from build123d import *

# Parameters (mm, degrees)
BOSS_EXTRUDE1_DEPTH            = 5
SKETCH3_W                      = 21
SKETCH3_H                      = 20
BOSS_EXTRUDE2_DEPTH            = 5
F_4_0MM_DOWEL_HOLE1_AT_2_COUNT = 2
F_4_0MM_DOWEL_HOLE1_AT_2_PITCH = 10
SKETCH15_W                     = 20
SKETCH15_H                     = 15
BOSS_EXTRUDE6_DEPTH            = 60
SKETCH16_W                     = 20
SKETCH16_H                     = 10
BOSS_EXTRUDE7_DEPTH            = 10


with BuildPart() as part:
    # Sketch2 → Boss-Extrude1 (new body)
    with BuildSketch(Plane(origin=(0, 0, 0), x_dir=(1, 0, 0), z_dir=(0, 1, 0))):
        Polygon((-80, -10), (-10, -10), (-10, -80), (10, -80), (10, -10), (80, -10), (80, 10), (10, 10), (10, 80), (-10, 80), (-10, 10), (-80, 10), align=None)
    extrude(amount=BOSS_EXTRUDE1_DEPTH)

    # Sketch3 → Boss-Extrude2 (add)
    with BuildSketch(Plane(origin=(0, 5, 0), x_dir=(1, 0, 0), z_dir=(0, 1, 0))):
        with Locations((-69.5, 0)):
            Rectangle(SKETCH3_W, SKETCH3_H)
    boss_extrude2 = extrude(amount=BOSS_EXTRUDE2_DEPTH)

    # Sketch5 → Ø4.0mm Dowel Hole1 (revolve, cut)
    with BuildSketch(Plane(origin=(-64.5, 10, 0), x_dir=(0, 0, 1), z_dir=(1, 0, 0))):
        Polygon((0, 0), (0, 118.830821238), (2, 117.6291), (2, 0), align=None)
    f_4_0mm_dowel_hole1 = revolve(axis=Axis((-64.5, 16.35, 0), (0, -1, 0)), mode=Mode.SUBTRACT)

    # Ø4.0mm Dowel Hole1 at 2: Ø4.0mm Dowel Hole1 ×2
    with Locations(*[(-i * F_4_0MM_DOWEL_HOLE1_AT_2_PITCH, 0, 0) for i in range(1, F_4_0MM_DOWEL_HOLE1_AT_2_COUNT)]):
        add(f_4_0mm_dowel_hole1, mode=Mode.SUBTRACT)

    # Mirror1: Boss-Extrude2, Ø4.0mm Dowel Hole1 across plane
    add(boss_extrude2.mirror(Plane(origin=(0, 0, 0), x_dir=(0, 0, 1), z_dir=(1, 0, 0))))
    add(f_4_0mm_dowel_hole1.mirror(Plane(origin=(0, 0, 0), x_dir=(0, 0, 1), z_dir=(1, 0, 0))), mode=Mode.SUBTRACT)

    # Mirror1 copy 1 sketch → Mirror1 copy 1 (revolve, cut)
    with BuildSketch(Plane(origin=(74.5, 10, 0), x_dir=(0, 0, 1), z_dir=(-1, 0, 0))):
        Polygon((0, 0), (0, -118.830821238), (2, -117.6291), (2, 0), align=None)
    revolve(axis=Axis((74.5, 16.35, 0), (0, 1, 0)), mode=Mode.SUBTRACT)

    # Sketch15 → Boss-Extrude6 (add)
    with BuildSketch(Plane(origin=(0, 5, 0), x_dir=(1, 0, 0), z_dir=(0, 1, 0))):
        with Locations((0, 48.5)):
            Rectangle(SKETCH15_W, SKETCH15_H)
        with Locations((0, -48.5)):
            Rectangle(SKETCH15_W, SKETCH15_H)
    extrude(amount=BOSS_EXTRUDE6_DEPTH)

    # Sketch16 → Boss-Extrude7 (add)
    with BuildSketch(Plane(origin=(0, 65, 0), x_dir=(1, 0, 0), z_dir=(0, 1, 0))):
        with Locations((0, 51)):
            Rectangle(SKETCH16_W, SKETCH16_H)
        with Locations((0, -51)):
            Rectangle(SKETCH16_W, SKETCH16_H)
    extrude(amount=BOSS_EXTRUDE7_DEPTH)


solid = part.part
Can you work these out from the model? Positions are in its coordinate system, mm. A direction names the side the tool comes from. Coordinates: 2 decimals unless noted, no trailing zeros. Order: outer loops, then holes, each group sorted by start corner. A loop starts at its lowest first (then second) coordinate and runs counter-clockwise, first axis right, second up. Notation, with made-up numbers: (40, 62) - (74, 62) arc R32 cw to (74, 98) - close; hole circle Ø5 at (74.5, -3). An arc over 180 degrees is marked (long way). Answer as a JSON object with one key per item and string values. Group by question number.
Q1. Will these pins go through, and if not, where does the flat tip stop? P1, Ø3, axis at x = -46.5, y = 6, coming from the +Z side; P2, Ø22, axis at x = -1, y = 30, coming from the -Z side; P3, Ø22, axis at x = -2, y = 53.5, coming from the +Z side.
Q2. We'd pull the mould along Z, two halves only. Please class faces 1 (the face through (0, 40, -56)), 2 (the face through (0, 65, -44)), 3 (the face through (0, 5, 68)): +Z half, -Z half, draft (parallel to the pull), parting line (faces both ways), or undercut.
Q3. Imagine slicing it at C-C (x = 64.5). Please give me the cut outline in (y, z), and give its area (3 significant figures).
Q4. Imagine slicing it at A-A (y = 8). Please give me the cut outline in (x, z), and give its area (3 significant figures).
Q5. I need wall thicknesses on line 1 (X direction, y = 4, z = 0); line 2 (X direction, y = 6, z = 0); line 3 (Y direction, x = -8.5, z = 73). Which ranges of each line are inside material? Lowest first, please. Write a range as from..to.
Q6. Imagine slicing it at D-D (z = 32). Please give me the cut outline in (x, y), and give its area (3 significant figures).
Q7. Imagine slicing it at B-B (y = 20). Please give me the cut outline in (x, z), and give its area (3 significant figures).
Q8. On a 3-axis mill with a long thin cutter (end or side, diameter ignored), from which of +Z, -Z, +X, -X, +Y, -Y can I reach the whole of each face in a straight line? I mean faces 4 (the face through (0, 35, -41)), 5 (the face through (-10, 29, -50)), 6 (the face through (59, 7, 0)), 7 (the face through (53, 4, -10)). Say none if no direction works.
Determined:
{
 "1": {"P1": "stops at z = 10", "P2": "stops at z = -56", "P3": "stops at z = 56"},
 "2": {"face 1": "-Z half", "face 2": "undercut", "face 3": "draft"},
 "3": {"outline": "(0, -10) - (10, -10) - (10, -2) - (0, -2) - close; (0, 2) - (10, 2) - (10, 10) - (0, 10) - close", "area": "160 mm2"},
 "4": {"outline": "(-80, -10) - (-59, -10) - (-59, 10) - (-80, 10) - close; (-10, -56) - (10, -56) - (10, -41) - (-10, -41) - close; (-10, 41) - (10, 41) - (10, 56) - (-10, 56) - close; (59, -10) - (80, -10) - (80, 10) - (59, 10) - close; hole circle Ø4 at (-74.5, 0); hole circle Ø4 at (-64.5, 0); hole circle Ø4 at (64.5, 0); hole circle Ø4 at (74.5, 0)", "area": "1,390 mm2"},
 "5": {"line 1": "x = -80..-76.5, -72.5..-66.5, -62.5..62.5, 66.5..72.5, 76.5..80", "line 2": "x = -80..-76.5, -72.5..-66.5, -62.5..-59, 59..62.5, 66.5..72.5, 76.5..80", "line 3": "y = 0..5"},
 "6": {"outline": "(-10, 0) - (10, 0) - (10, 5) - (-10, 5) - close", "area": "100 mm2"},
 "7": {"outline": "(-10, -56) - (10, -56) - (10, -41) - (-10, -41) - close; (-10, 41) - (10, 41) - (10, 56) - (-10, 56) - close", "area": "600 mm2"},
 "8": {"face 4": "+X, -X, +Y", "face 5": "-Z, -X, +Y, -Y", "face 6": "+Z, -Z, +Y", "face 7": "-Z, +X, +Y, -Y"}
}
